Source: CAD feature listing. Evaluate the final solid. Frame: model axes, mm. A direction names the side the tool comes from. Give positions to 0.01 mm unless a question says otherwise; leave off trailing zeros. Write each loop counter-clockwise with the first axis right and the second up, starting at its lowest first coordinate (ties: lowest second). Pieces come first, ordered by that corner, then holes.
```python
from build123d import *

# Parameters (mm, degrees)
SKETCH1_W           = 57.15
SKETCH1_H           = 50.8
BOSS_EXTRUDE1_DEPTH = 4.800000052
SKETCH3_W           = 9.600000104
SKETCH3_H           = 16.933333334
CUT_EXTRUDE2_DEPTH  = 48.255810933
SKETCH7_R           = 17.849200014
CUT_EXTRUDE6_DEPTH  = 100.442088012
SKETCH4_W           = 4.500000144
SKETCH4_H           = 8.466666666
SKETCH4_H_2         = 8.357391871
CUT_EXTRUDE7_DEPTH  = 48.255810933
SKETCH8_R           = 17.849200014
CUT_EXTRUDE8_DEPTH  = 100.528553706


with BuildPart() as part:
    # Sketch1 → Boss-Extrude1 (new body)
    with BuildSketch(Plane.XY):
        with Locations((-10.098235381, 1.329244875)):
            Rectangle(SKETCH1_W, SKETCH1_H)
    extrude(amount=BOSS_EXTRUDE1_DEPTH)

    # Sketch3 → Cut-Extrude2 (cut, through all)
    with BuildSketch(Plane.XY.offset(4.800000052)):
        with Locations((13.676764567, 1.329244875)):
            Rectangle(SKETCH3_W, SKETCH3_H)
    extrude(amount=-CUT_EXTRUDE2_DEPTH, mode=Mode.SUBTRACT)

    # Sketch7 → Cut-Extrude6 (cut, through all)
    with BuildSketch(Plane(origin=(21.96927249, 54.594199632, 4.800000052), x_dir=(0.8370756248818486, 0.5470871943563135, 0), z_dir=(0, 0, 1))):
        with Locations(Location((-61.009273933, -23.888925268, 0), (0, 0, 326.832589089))):
            Circle(SKETCH7_R)
    extrude(amount=-CUT_EXTRUDE6_DEPTH, mode=Mode.SUBTRACT)

    # Sketch4 → Cut-Extrude7 (cut, through all)
    with BuildSketch(Plane(origin=(0, 0, 0), x_dir=(-1, 0, 0), z_dir=(0, 0, -1))):
        with Locations((-11.126764587, 14.029244875)):
            Rectangle(SKETCH4_W, SKETCH4_H)
        with Locations((-11.126764587, -19.89205919)):
            Rectangle(SKETCH4_W, SKETCH4_H_2)
    extrude(amount=-CUT_EXTRUDE7_DEPTH, mode=Mode.SUBTRACT)

    # Sketch8 → Cut-Extrude8 (cut, through all)
    with BuildSketch(Plane(origin=(21.96927249, 54.703474427, 0), x_dir=(0, -1, 0), z_dir=(0, 0, -1))):
        with Locations((53.374229552, 38.000051)):
            Circle(SKETCH8_R)
    extrude(amount=-CUT_EXTRUDE8_DEPTH, mode=Mode.SUBTRACT)


solid = part.part
```
1. Line query: L1, parallel to Y at x = 14, z = 0.6; L2, parallel to Y at x = 13, z = 2.8; L3, parallel to X at y = 16.5, z = 4.4. Output: solid intervals per line, ascending.
2. Access query for faces 1 (the flat face through (13.377, -20, 2)), 2 (the flat face through (13.377, 14, 2)), 3 (the flat face through (-15, -24.071, 2)), 4 (the flat face through (16, 9.796, 2)). Directions: +Z, -Z, +X, -X, +Y, -Y. A direction counts if a zero-diameter tool reaches every point of the face in a straight line with its end or side. Return the directions, or none.
3. Contact query for flat-ended pins moving along their axis: P1, Ø2, axis at x = -31.5, y = -16, coming from the -Z side; P2, Ø1.4, axis at x = 11, z = 2.5, coming from the -Y side; P3, Ø2.5, axis at y = 7, z = 2, coming from the +X side. Output: stop coordinate, or through.
4. Cut plane B-B, the plane x = -28. Return the cut outline in (y, z).
5. Cut plane C-C, the plane z = 4. Return the cut outline in (x, y), then the cut area to 3 significant figures.
6. Cut plane A-A, the plane y = -19. Return the cut outline in (x, z), then the cut area to 3 significant figures.
7. Mould query, pull axis X, two halves, no side actions, for faces 5 (the flat face through (18.477, -16, 2)), 6 (the flat face through (11, 18.263, 2)), 7 (the flat face through (14, -7.137, 2)). Classes: +X half, -X half, draft (parallel to the pull), parting line (faces both ways), or undercut.
Response values:
1. L1: y = -24.07 to -7.14, 9.8 to 26.73
1. L2: y = -15.71 to -7.14, 18.26 to 26.73
1. L3: x = -38.67 to -25.44, -6.63 to 8.88, 13.38 to 18.48
2. face 1: +Z, -Z, -Y
2. face 2: +Z, -Z
2. face 3: +Z, -Z, +X, -X, -Y
2. face 4: +Z, -Z, +X
3. P1: stops at z = 0
3. P2: stops at y = -15.71
3. P3: stops at x = 8.88
4. outline: (-24.07, 0) - (-12.02, 0) - (-12.02, 4.8) - (-24.07, 4.8) - close; (14.57, 0) - (26.73, 0) - (26.73, 4.8) - (14.57, 4.8) - close
5. outline: (-38.67, -24.07) - (8.88, -24.07) - (8.88, -15.71) - (13.38, -15.71) - (13.38, -24.07) - (18.48, -24.07) - (18.48, -7.14) - (8.88, -7.14) - (8.88, 18.26) - (13.38, 18.26) - (13.38, 9.8) - (18.48, 9.8) - (18.48, 26.73) - (-38.67, 26.73) - close; hole (-33.88, 1.27) arc R17.85 ccw (long way) to (1.82, 1.27) arc R17.85 ccw (long way) to start
5. area: 1,660 mm2
6. outline: (-38.67, 0) - (8.88, 0) - (8.88, 4.8) - (-38.67, 4.8) - close; (13.38, 0) - (18.48, 0) - (18.48, 4.8) - (13.38, 4.8) - close
6. area: 253 mm2
7. face 5: +X half
7. face 6: undercut
7. face 7: draft
